Verification items for the finished model (mm, model axes). A direction names the side the tool comes from. Coordinates: 2 decimals unless noted, no trailing zeros. Order: outer loops, then holes, each group sorted by start corner. A loop starts at its lowest first (then second) coordinate and runs counter-clockwise, first axis right, second up. Notation, with made-up numbers: M -7,73.25 L 25,73.25 A18 cw 25,103.25 Z; hole C -7.5,78.25 d6. An arc over 180 degrees is marked long. Write item = value, one per line.
Autodesk Inventor part; units mm, degrees
ref_plane "YZ Plane" through (0, 0, 0) normal (1, 0, 0) x (0, 1, 0)
ref_plane "XZ Plane" through (0, 0, 0) normal (0, 1, 0) x (-1, 0, 0)
ref_plane "XY Plane" through (0, 0, 0) normal (0, 0, 1) x (1, 0, 0)
sketch "Sketch6" plane through (0, 0, 0) normal (0, 0, 1) x (1, 0, 0)
  line L0 (18, 18) -> (-18, 18)
  line L1 (-18, 18) -> (-18, -18)
  line L2 (-18, -18) -> (18, -18)
  line L3 (18, -18) -> (18, 18)
  line L4 (18, 18) -> (-18, -18) construction
  circle A0 centre (0, -34) radius 5.55
  circle A1 centre (35, 20) radius 5.55
  circle A2 centre (-35, 20) radius 5.55
  line L5 (35, 20) -> (-35, 20) construction
  line L6 (-35, 20) -> (0, -34) construction
  line L7 (0, -34) -> (35, 20) construction
  line L8 (0, 18) -> (0, -18) construction
  line L9 (-47.5046, 28) -> (47.5046, 28)
  line L10 (-18, 18) -> (23.6569, -23.6569) construction
  line L11 (18, 18) -> (-23.6569, -23.6569) construction
  line L12 (47.5046, 28) -> (23.6569, -23.6569)
  line L13 (23.6569, -23.6569) -> (0, -44.709)
  line L14 (0, -44.709) -> (-23.6569, -23.6569)
  line L15 (-47.5046, 28) -> (-23.6569, -23.6569)
  line L16 (-35, 20) -> (-42.2633, 16.6468) construction
  line L17 (0, -34) -> (-5.3183, -39.9763) construction
  point P0 (0, 0)
  point P1 (0, 0)
  point P2 (60, 0)
  point P3 (0, 28)
  point P4 (0, 0)
  dimension "d30" = 36
  dimension "d31" = 36
  dimension "d33" = 11.1
  dimension "d37" = 64.3506
  dimension "d52" = 70
  dimension "d53" = 8
  dimension "d54" = 20
  dimension "d57" = 8
  dimension "d59" = 8
  dimension "d60" = 95.0092
  dimension "d61" = 54
  dimension "d62" = 8
  dimension "d63" = 8
  dimension "d64" = 10
extrude "Plate3" add sketch "Sketch6" along normal blind 3
fillet "Corner Round2" radius 6 5 edges at (-47.5046, 28, 1.5) (47.5046, 28, 1.5) (0, -44.709, 1.5) (-23.6569, -23.6569, 1.5) (23.6569, -23.6569, 1.5)
equation "\"d41\" = Thickness"
equation "\"BendReliefWidth\" = Thickness"
equation "\"BendReliefDepth\" = 0.5 * Thickness"
equation "\"CornerReliefSize\" = 4 * Thickness"
equation "\"MinimumRemnant\" = 2 * Thickness"
equation "\"TransitionRadius\" = BendRadius"
equation "\"JacobiRadiusSize\" = BendRadius"
equation "\"GapSize\" = Thickness"
properties part number "DSB-507 beam flange" material "Stainless Steel"
Item 1: Gauge pin test, flat ends, axial feed: pin 1 (10 mm diameter, centred on x = -35, y = 20, fed in from +Z); pin 2 (1.5 mm diameter, centred on y = 1, z = 2, fed in from +X); pin 3 (1.5 mm diameter, centred on x = -4, z = 2, fed in from -Y); pin 4 (1.5 mm diameter, centred on y = -4.5, z = 1.5, fed in from -X). Record the tip position at first contact, or that the pin passes through.
Report:
pin_1 = through
pin_2 = 35.39
pin_3 = -41.72
pin_4 = -32.85
Item 2: Tool access check on faces 1 (the flat face through (0, 18, 1)), 2 (the cylindrical face through (-43.134, 25.304, 1.521)). Record the directions out of +Z, -Z, +X, -X, +Y, -Y that give a thin tool (end or side, any length) a straight path to the whole face; none if there is none.
Report:
face_1 = +Z, -Z
face_2 = +Z, -Z, -X
Item 3: Sectioned sample at C-C, the plane x = 35. Enter the section's corners in (y, z), then the cut area to 3 significant figures.
Report:
outline = M 0.91,0 L 14.45,0 L 14.45,3 L 0.91,3 Z; M 25.55,0 L 28,0 L 28,3 L 25.55,3 Z
area = 48.0 mm^2
Item 4: Scan lines: L1, parallel to Y at x = 0, z = 1.8; L2, parallel to X at y = 16.5, z = 0.3; L3, parallel to X at y = -10.5, z = 1.15. Record each from-to range of solid material in increasing order. Write a range as from..to.
Report:
L1 = -42.68..-39.55, -28.45..-18, 18..28
L2 = -42.2..-39.31, -30.69..-18, 18..30.69, 39.31..42.2
L3 = -29.73..-18, 18..29.73
Item 5: Sectioned sample at A-A, the plane x = 0. Enter the section's corners in (y, z).
Report:
outline = M -42.68,0 L -39.55,0 L -39.55,3 L -42.68,3 Z; M -28.45,0 L -18,0 L -18,3 L -28.45,3 Z; M 18,0 L 28,0 L 28,3 L 18,3 Z
Item 6: Sectioned sample at D-D, the plane y = -6.5. Enter the section's corners in (x, z), then the cut area to 3 significant figures.
Report:
outline = M -31.58,0 L -18,0 L -18,3 L -31.58,3 Z; M 18,0 L 31.58,0 L 31.58,3 L 18,3 Z
area = 81.5 mm^2
Item 7: Release check for a two-part mould opening along Y. For faces 3 (the flat face through (18, 0, 1)), 4 (the flat face through (34.013, -1.224, 1.479)), 5 (the cylindrical face through (34.278, 14.497, 1.479)), 6 (the flat face through (19, 1, 3)) record: pulls with the +Y half, pulls with the -Y half, needs draft (parallel to the pull), parting line crosses it, or undercut.
Report:
face_3 = undercut
face_4 = pulls with the -Y half
face_5 = undercut
face_6 = needs draft
Item 8: Sectioned sample at B-B, the plane z = 1.9. Enter the section's corners in (x, y).
Report:
outline = M -43.57,19.49 L -24.18,-22.52 A6 ccw -22.72,-24.49 L -3.99,-41.16 A6 ccw 3.99,-41.16 L 22.72,-24.49 A6 ccw 24.18,-22.52 L 43.57,19.49 A6 ccw 38.13,28 L -38.13,28 A6 ccw Z; hole C -35,20 d11.1; hole M -18,-18 L 18,-18 L 18,18 L -18,18 Z; hole C 0,-34 d11.1; hole C 35,20 d11.1
